Part model, mm, in its own coordinate system. A direction names the side the tool comes from. Coordinates: 2 decimals unless noted, no trailing zeros. Loops run counter-clockwise (first coordinate to the right, second up) from the corner with the lowest first, then second, coordinate; pieces in that order, holes last. Notation, with made-up numbers: (-9, 4) - (10, 4) arc R24 cw to (10, 28) - close; hole circle Ø1 at (37.25, 57.5). An arc over 180 degrees is marked (long way). Use a Markdown table: item, result. Add a question column.
1. Wall check: probe 1 along Z at (x, y) = (46, -23); probe 2 along Z at (x, y) = (25, -7); probe 3 along Y at (x, z) = (-15, 6). Give the ranges that are in metal, low to high. Write a range as [from, to].
2. Band-saw the part on B-B, the plane z = 0. Give the cut face in (x, y), plus the area to 3 significant figures.
3. Drop flat-ended pins along their axis: pin 1 (8 mm diameter, centred on x = -35, y = -64, fed in from -Z); pin 2 (2 mm diameter, centred on x = 27, y = -39.5, fed in from +Z). Give the stop position or say it passes through.
4. Band-saw the part on A-A, the plane x = 0. Give the cut face in (y, z).
5. 3-axis set-ups, long thin cutter, end or side, ignore diameter. For faces 1 (the flat face through (0, -22, 80)), 2 (the cylindrical face through (-3.252, -36.587, 64.79)), 3 (the cylindrical face through (-3.252, -10.286, -64.79)): which of +Z, -Z, +X, -X, +Y, -Y reach the whole face in a straight line?
6. Band-saw the part on D-D, the plane y = -61.5. Give the cut face in (x, z).
7. Band-saw the part on C-C, the plane x = -39. Give the cut face in (y, z), plus the area to 3 significant figures.
from build123d import *

# Parameters (mm, degrees)
F0_W     = 100
F0_H     = 100
F1_DEPTH = 100
F2_R     = 15
F3_DEPTH = 30
F4_R     = 15
F5_DEPTH = 30
F7_D     = 30


with BuildPart() as f1:
    # F0 (on Front) → F1 (new body)
    with BuildSketch(Plane.XZ):
        Rectangle(F0_W, F0_H)
    extrude(amount=F1_DEPTH)

    # F2 (on face) → F3 (join)
    with BuildSketch(Plane.XY.offset(50)):
        with Locations((0, -21.943816)):
            Circle(F2_R)
    extrude(amount=F3_DEPTH)

    # F4 (on face) → F5 (join)
    with BuildSketch(Plane(origin=(0, 0, -50), x_dir=(1, 0, 0), z_dir=(0, 0, -1))):
        with Locations((0, 24.92946)):
            Circle(F4_R)
    extrude(amount=F5_DEPTH)

    # F7 (through all)
    with Locations(Plane.YZ.offset(50)):
        with Locations((-23.007467, 0)):
            Hole(F7_D / 2)


solid = f1.part
Geometry check:
| question | item | result |
|---|---|---|
| 1 | probe 1 | z = [-50, -15], [15, 50] |
| 1 | probe 2 | z = [-50, 50] |
| 1 | probe 3 | y = [-100, -36.76], [-9.26, 0] |
| 2 | outline | (-50, -100) - (50, -100) - (50, -38.01) - (-50, -38.01) - close; (-50, -8.01) - (50, -8.01) - (50, 0) - (-50, 0) - close |
| 2 | area | 7,000 mm^2 |
| 3 | pin 1 | stops at z = -50 |
| 3 | pin 2 | stops at z = 50 |
| 4 | outline | (-100, -50) - (-39.93, -50) - (-39.93, -80) - (-9.93, -80) - (-9.93, -50) - (0, -50) - (0, 50) - (-6.94, 50) - (-6.94, 80) - (-36.94, 80) - (-36.94, 50) - (-100, 50) - close; hole circle Ø30 at (-23.01, 0) |
| 5 | face 1 | +Z, +X, -X, +Y, -Y |
| 5 | face 2 | +Z |
| 5 | face 3 | -Z |
| 6 | outline | (-50, -50) - (50, -50) - (50, 50) - (-50, 50) - close |
| 7 | outline | (-100, -50) - (0, -50) - (0, 50) - (-100, 50) - close; hole circle Ø30 at (-23.01, 0) |
| 7 | area | 9,290 mm^2 |
